The model under review builds one solid part; all positions refer to its coordinate system, in mm. A direction names the side the tool comes from. Round coordinates to 2 decimals unless told otherwise and drop trailing zeros. Loops run counter-clockwise (first coordinate to the right, second up) from the corner with the lowest first, then second, coordinate; pieces in that order, holes last. Notation, with made-up numbers: M 20,44 L 64,44 A13 ccw 64,48 Z; hole C 82,61.25 d9. An arc over 180 degrees is marked long. Return JSON: item names as keys, results as strings. Group by question number.
Q1. For faces 5 (the face through (-40.51, -33.85, 14.86)), 6 (the face through (-103.65, 96.99, 12.68)), 7 (the face through (36.65, -87.99, 14.86)), 8 (the face through (-84, -40, 30)), list the 3-axis set-ups (+Z, -Z, +X, -X, +Y, -Y) from which the entire face can be reached by the end or side of a thin tool; tool diameter is ignored.
Q2. Consider section C-C (z = 47). State the section outline as (x, y) points.
Q3. Draft analysis for pull direction Y (two halves, no side actions). For faces 1 (the face through (46, 24, 25)), 2 (the face through (-47, -33, 25)), 3 (the face through (103.49, -97.15, 12.68)), 4 (the face through (-50.305, 46.08, 14.86)), state which applies: pulls with the +Y half, pulls with the -Y half, needs draft (parallel to the pull), parting line crosses it, or undercut.
Q4. Clearance check with flat-ended pins moving along their axes: pin 1 Ø1 at (x, z) = (-30.5, 99.5) entering from -Y; pin 2 Ø12 at (x, y) = (-7.5, -50) entering from +Z; pin 3 Ø24.5 at (x, y) = (-71.5, -66) entering from +Z; pin 4 Ø18 at (x, y) = (-76.5, -70) entering from -Z. State where each tip first meets the part, or that it passes through.
Q5. To check wall thickness, follow line 1 along Y through (x, z) = (-76.5, 28) (3 decimals); line 2 along Y through (x, z) = (-76.5, 6.75) (3 decimals); line 3 along Y through (x, z) = (-48.5, 95). State the ranges of each line that lie inside material, in increasing order.
Q6. Consider section A-A (y = -70). State the section outline as (x, z) points (1 decimal).
Q7. Consider section B-B (x = -76.5). State the section outline as (y, z) points (3 decimals), and give its area (3 significant figures).
Q8. Consider section D-D (y = 7). State the section outline as (x, z) points.
from build123d import *

# Parameters (mm, degrees)
F0_W            = 213
F0_H            = 200
F1_DEPTH        = 25
F2_W            = 60
F2_H            = 60
F3_DEPTH        = 10
F4_R            = 10
F5_R            = 15
F6_DEPTH        = 20
F7_DEPTH        = 70
F8_R            = 10
F10_DEPTH       = 120
F11_DEPTH       = 120
F12_SIZE        = 2
F14_DEPTH       = 120
F15_DEPTH       = 120
F16_SIZE        = 2
F18_D           = 14.75
F18_CBORE_D     = 22.25
F18_CBORE_DEPTH = 14
F19_SIZE        = 2
F20_SIZE        = 2


with BuildPart() as f1:
    # F0 (on Top) → F1 (new body)
    with BuildSketch(Plane.XY):
        Rectangle(F0_W, F0_H)
    extrude(amount=F1_DEPTH)

    # F2 (on face) → F3 (join)
    with BuildSketch(Plane.XY.offset(25)):
        with Locations((-76.5, -70)):
            Rectangle(F2_W, F2_H)
    extrude(amount=F3_DEPTH)

    # F4
    f4_edges = [f1.edges().sort_by_distance(p)[0] for p in [
        (-106.5, -100, 17.5),
        (106.5, -100, 12.5),
        (106.5, 100, 12.5),
        (-106.5, 100, 12.5),
    ]]
    fillet(f4_edges, radius=F4_R)

    # F5
    f5_edges = [f1.edges().sort_by_distance(p)[0] for p in [
        (-46.5, -40, 30),
    ]]
    fillet(f5_edges, radius=F5_R)

    # F2 (on face) → F6 (cut)
    with BuildSketch(Plane.XY.offset(25)):
        with BuildLine():
            Line((-48.3758740693, 48.0959181604), (-97.5, 48.0959181604))
            Line((-97.5, 48.0959181604), (-97.5, -31))
            Line((-97.5, -31), (-37.5, -31))
            Line((-37.5, -31), (-37.5, -91))
            Line((-37.5, -91), (39.5, -91))
            Line((39.5, -91), (39.5, -41.445053726))
            ThreePointArc((39.5, -41.445053726), (-17.8631347732, -9.8501114582), (-48.3758740693, 48.0959181604))
        make_face()
    extrude(amount=-F6_DEPTH, mode=Mode.SUBTRACT)

    # F2 (on face) → F7 (join)
    with BuildSketch(Plane.XY.offset(25)):
        with BuildLine():
            Line((48.5, -33.9230484541), (48.5, -100))
            Line((48.5, -100), (63.5, -100))
            Line((63.5, -100), (63.5, -20))
            ThreePointArc((63.5, -20), (-0.1396103068, 6.3603896932), (-26.5, 70))
            Line((-26.5, 70), (-106.5, 70))
            Line((-106.5, 70), (-106.5, 57.0959181604))
            Line((-106.5, 57.0959181604), (-40.7040530492, 57.0959181604))
            ThreePointArc((-40.7040530492, 57.0959181604), (-11.4900969244, -3.4947982055), (48.5, -33.9230484541))
        make_face()
    extrude(amount=F7_DEPTH)

    # F8
    f8_edges = [f1.edges().sort_by_distance(p)[0] for p in [
        (-48.375874, 48.095918, 15),
        (39.5, -41.445054, 15),
        (-37.5, -31, 15),
        (-97.5, 48.095918, 15),
        (39.5, -91, 15),
        (-37.5, -91, 15),
        (-97.5, -31, 15),
    ]]
    fillet(f8_edges, radius=F8_R)

    # F9 (on face) → F10 (cut)
    with BuildSketch(Plane(origin=(-106.5, 0, 0), x_dir=(0, -1, 0), z_dir=(-1, 0, 0))):
        with BuildLine():
            ThreePointArc((-43.0479590802, 95), (-75.5476082656, 111.621023417), (-70, 75.5418097458))
            Line((-70, 75.5418097458), (-70, 95))
            Line((-70, 95), (-57.0959181604, 95))
            Line((-57.0959181604, 95), (-57.0959181604, 75.5418097458))
            ThreePointArc((-57.0959181604, 75.5418097458), (-46.9269356632, 83.0003508146), (-43.0479590802, 95))
        make_face()
        with BuildLine():
            Line((-70, 95), (-70, 75.5418097458))
            ThreePointArc((-70, 75.5418097458), (-63.5479590802, 74.5), (-57.0959181604, 75.5418097458))
            Line((-57.0959181604, 75.5418097458), (-57.0959181604, 95))
            Line((-57.0959181604, 95), (-70, 95))
        make_face()
        with BuildLine():
            ThreePointArc((-57.0959181604, 60.09124511), (-36.2597065468, 72.2931447868), (-28.0479590802, 95))
            ThreePointArc((-28.0479590802, 95), (-86.2548142934, 122.2882525334), (-70, 60.09124511))
            Line((-70, 60.09124511), (-70, 75.5418097458))
            ThreePointArc((-70, 75.5418097458), (-75.5476082656, 111.621023417), (-43.0479590802, 95))
            ThreePointArc((-43.0479590802, 95), (-46.9269356632, 83.0003508146), (-57.0959181604, 75.5418097458))
            Line((-57.0959181604, 75.5418097458), (-57.0959181604, 60.09124511))
        make_face()
    extrude(amount=-F10_DEPTH, mode=Mode.SUBTRACT)

    # F9 (on face) → F11 (join)
    with BuildSketch(Plane(origin=(-106.5, 0, 0), x_dir=(0, -1, 0), z_dir=(-1, 0, 0))):
        with BuildLine():
            ThreePointArc((-57.0959181604, 60.09124511), (-36.2597065468, 72.2931447868), (-28.0479590802, 95))
            ThreePointArc((-28.0479590802, 95), (-86.2548142934, 122.2882525334), (-70, 60.09124511))
            Line((-70, 60.09124511), (-70, 75.5418097458))
            ThreePointArc((-70, 75.5418097458), (-75.5476082656, 111.621023417), (-43.0479590802, 95))
            ThreePointArc((-43.0479590802, 95), (-46.9269356632, 83.0003508146), (-57.0959181604, 75.5418097458))
            Line((-57.0959181604, 75.5418097458), (-57.0959181604, 60.09124511))
        make_face()
        with BuildLine():
            Line((-70, 75.5418097458), (-70, 60.09124511))
            ThreePointArc((-70, 60.09124511), (-63.5479590802, 59.5), (-57.0959181604, 60.09124511))
            Line((-57.0959181604, 60.09124511), (-57.0959181604, 75.5418097458))
            ThreePointArc((-57.0959181604, 75.5418097458), (-63.5479590802, 74.5), (-70, 75.5418097458))
        make_face()
    extrude(amount=-F11_DEPTH)

    # F12
    f12_edges = [f1.edges().sort_by_distance(p)[0] for p in [
        (-106.5, 84.047959, 95),
    ]]
    chamfer(f12_edges, length=F12_SIZE)

    # F13 (on face) → F14 (cut)
    with BuildSketch(Plane.XZ.offset(100)):
        with BuildLine():
            ThreePointArc((76.5, 95), (44.4566036194, 111.9410743461), (48.5, 75.9212159717))
            Line((48.5, 75.9212159717), (48.5, 95))
            Line((48.5, 95), (63.5, 95))
            Line((63.5, 95), (63.5, 75.9212159717))
            ThreePointArc((63.5, 75.9212159717), (72.9410743461, 83.4566036194), (76.5, 95))
        make_face()
        with BuildLine():
            Line((48.5, 95), (48.5, 75.9212159717))
            ThreePointArc((48.5, 75.9212159717), (56, 74.5), (63.5, 75.9212159717))
            Line((63.5, 75.9212159717), (63.5, 95))
            Line((63.5, 95), (48.5, 95))
        make_face()
    extrude(amount=-F14_DEPTH, mode=Mode.SUBTRACT)

    # F13 (on face) → F15 (join)
    with BuildSketch(Plane.XZ.offset(100)):
        with BuildLine():
            ThreePointArc((63.5, 57.4073514866), (85.6391503948, 70.6899612068), (94.3335, 95))
            ThreePointArc((94.3335, 95), (31.6899612068, 124.6391503948), (48.5, 57.4073514866))
            Line((48.5, 57.4073514866), (48.5, 75.9212159717))
            ThreePointArc((48.5, 75.9212159717), (44.4566036194, 111.9410743461), (76.5, 95))
            ThreePointArc((76.5, 95), (72.9410743461, 83.4566036194), (63.5, 75.9212159717))
            Line((63.5, 75.9212159717), (63.5, 57.4073514866))
        make_face()
        with BuildLine():
            Line((48.5, 75.9212159717), (48.5, 57.4073514866))
            ThreePointArc((48.5, 57.4073514866), (56, 56.6665), (63.5, 57.4073514866))
            Line((63.5, 57.4073514866), (63.5, 75.9212159717))
            ThreePointArc((63.5, 75.9212159717), (56, 74.5), (48.5, 75.9212159717))
        make_face()
    extrude(amount=-F15_DEPTH)

    # F16
    f16_edges = [f1.edges().sort_by_distance(p)[0] for p in [
        (35.5, -100, 95),
    ]]
    chamfer(f16_edges, length=F16_SIZE)

    # F18 (through all)
    with Locations(Plane.XY.offset(35)):
        with Locations((-76.5, -70)):
            CounterBoreHole(F18_D / 2, F18_CBORE_D / 2, F18_CBORE_DEPTH)

    # F19
    f19_edges = [f1.edges().sort_by_distance(p)[0] for p in [
        (35.5, 20, 95),
    ]]
    chamfer(f19_edges, length=F19_SIZE)

    # F20
    f20_edges = [f1.edges().sort_by_distance(p)[0] for p in [
        (13.5, 84.047959, 95),
    ]]
    chamfer(f20_edges, length=F20_SIZE)


solid = f1.part
Values:
{
 "1": {"face 5": "+Z", "face 6": "-Z, -X, +Y", "face 7": "none", "face 8": "+Z, -X"},
 "2": {"outline": "M -106.5,57.1 L -40.7,57.1 A105 ccw 48.5,-33.92 L 48.5,-100 L 63.5,-100 L 63.5,-20 A90 cw -26.5,70 L -106.5,70 Z"},
 "3": {"face 1": "needs draft", "face 2": "undercut", "face 3": "pulls with the -Y half", "face 4": "undercut"},
 "4": {"pin 1": "stops at y = 28.27", "pin 2": "stops at z = 5", "pin 3": "stops at z = 35", "pin 4": "stops at z = 0"},
 "5": {"line 1": "y = -100 to -81.125, -58.875 to -40, 57.096 to 70", "line 2": "y = -100 to -77.375, -62.625 to -31, 48.096 to 100", "line 3": "y = 28.05 to 43.05, 84.05 to 99.05"},
 "6": {"outline": "M -106.5,0 L -83.9,0 L -83.9,21 L -87.6,21 L -87.6,35 L -106.5,35 Z; M -69.1,0 L 106.5,0 L 106.5,25 L 63.5,25 L 63.5,57.4 A38.3 ccw long 48.5,57.4 L 48.5,25 L 39.5,25 L 39.5,5 L -37.5,5 L -37.5,25 L -46.5,25 L -46.5,35 L -65.4,35 L -65.4,21 L -69.1,21 Z; hole C 56,95 d41"},
 "7": {"outline": "M -100,0 L -77.375,0 L -77.375,21 L -81.125,21 L -81.125,35 L -100,35 Z; M -62.625,0 L 100,0 L 100,25 L 70,25 L 70,60.091 A35.5 ccw long 57.096,60.091 L 57.096,25 L 48.096,25 L 48.096,5 L -31,5 L -31,25 L -40,25 L -40,35 L -58.875,35 L -58.875,21 L -62.625,21 Z; hole C 63.548,95 d41", "area": "6,480 mm2"},
 "8": {"outline": "M -106.5,0 L 106.5,0 L 106.5,25 L -0.77,25 L -0.77,95 L -20.5,95 L -20.5,25 L -31.51,25 L -31.51,5 L -97.5,5 L -97.5,25 L -106.5,25 Z; C 56,95 d76.67; hole C 56,95 d41"}
}
